Verification items for the finished model (mm, model axes). Face numbers are marked on the shaded views. A direction names the side the tool comes from. Coordinates: 2 decimals unless noted, no trailing zeros. Order: outer loops, then holes, each group sorted by start corner. A loop starts at its lowest first (then second) coordinate and runs counter-clockwise, first axis right, second up. Notation, with made-up numbers: M 20.5,-12 L 78.5,-12 A22 cw 78.5,22 Z; hole C 1,-1 d7. An arc over 180 degrees is marked long. Return JSON: item names as keys, results as strings. Group by question number.
1. Section check D-D, the plane z = 25. Record the cut outline in (x, y).
2. Material ranges on line 1 along Z through (x, y) = (-10, 3.25); line 2 along Z through (x, y) = (63, 23.5); line 3 along Z through (x, y) = (-51, 9.25), recorded low to high.
3. Set-up check for the marked faces 1 and 2: record each of +Z, -Z, +X, -X, +Y, -Y from which the full face is reachable in a straight line by a thin tool's end or side.
4. Gauge pin test, flat end, axial feed: pin 1 (12 mm diameter, centred on x = -0.5, z = -28.5, fed in from +Y). Record the tip position at first contact, or that the pin passes through.
5. Section check C-C, the plane y = 6.75. Record the cut outline in (x, z), plus the area to 3 significant figures.
6. Mould release check, pull along X, two halves, no side actions. Record for the marked faces 3, 4 and 5: +X half, -X half, draft (parallel to the pull), parting line (faces both ways), or undercut.
7. Section check B-B, the plane z = -16. Record the cut outline in (x, y).
8. Section check A-A, the plane x = 45. Record the cut outline in (y, z).
```python
from build123d import *

# Parameters (mm, degrees)
SKETCH1_W                      = 142
SKETCH1_H                      = 82
BOSS_EXTRUDE1_DEPTH            = 30
SKETCH3_W                      = 130
SKETCH3_H                      = 70
CUT_EXTRUDE1_DEPTH             = 25
FILLET1_R                      = 5
M3_CLEARANCE_HOLE1_D           = 3.2
M3_CLEARANCE_HOLE1_CSINK_D     = 3.25
M3_CLEARANCE_HOLE1_CSINK_ANGLE = 90
CUT_EXTRUDE2_REACH             = 7
CUT_EXTRUDE3_DEPTH             = 143


with BuildPart() as part:
    # Sketch1 → Boss-Extrude1 (new body)
    with BuildSketch(Plane(origin=(0, 0, 0), x_dir=(1, 0, 0), z_dir=(0, 1, 0))):
        Rectangle(SKETCH1_W, SKETCH1_H)
    extrude(amount=BOSS_EXTRUDE1_DEPTH)

    # Sketch3 → Cut-Extrude1 (cut)
    with BuildSketch(Plane(origin=(0, 30, 0), x_dir=(1, 0, 0), z_dir=(0, 1, 0))):
        Rectangle(SKETCH3_W, SKETCH3_H)
    extrude(amount=-CUT_EXTRUDE1_DEPTH, mode=Mode.SUBTRACT)

    # Fillet1
    fillet1_edges = [part.edges().sort_by_distance(p)[0] for p in [
        (71, 15, 41),
        (-71, 15, 41),
        (-71, 15, -41),
        (71, 15, -41),
    ]]
    fillet(fillet1_edges, radius=FILLET1_R)

    # M3 Clearance Hole1 (through all)
    with Locations(Plane(origin=(0, 30, 0), x_dir=(1, 0, 0), z_dir=(0, 1, 0))):
        with Locations((63, -38), (63, 38), (-63, 38), (-63, -38)):
            CounterSinkHole(M3_CLEARANCE_HOLE1_D / 2, M3_CLEARANCE_HOLE1_CSINK_D / 2, counter_sink_angle=M3_CLEARANCE_HOLE1_CSINK_ANGLE)

    # Sketch6 → Cut-Extrude2 (cut, up to next)
    with BuildSketch(Plane(origin=(0, 5, 0), x_dir=(1, 0, 0), z_dir=(0, 1, 0)), mode=Mode.PRIVATE) as cut_extrude2_sk1:
        with BuildLine():
            Line((52.5, -30), (-52.5, -30))
            ThreePointArc((-52.5, -30), (-57.5, -25), (-52.5, -20))
            Line((-52.5, -20), (52.5, -20))
            ThreePointArc((52.5, -20), (57.5, -25), (52.5, -30))
        make_face()
    cut_extrude2_tool1 = extrude(cut_extrude2_sk1.sketch, amount=-CUT_EXTRUDE2_REACH, mode=Mode.PRIVATE) & part.part
    add(cut_extrude2_tool1.solids().sort_by_distance((0, 5, 25))[0], mode=Mode.SUBTRACT)
    # Sketch6 → Cut-Extrude2 (cut, up to next)
    with BuildSketch(Plane(origin=(0, 5, 0), x_dir=(1, 0, 0), z_dir=(0, 1, 0)), mode=Mode.PRIVATE) as cut_extrude2_sk2:
        with BuildLine():
            Line((52.5, 20), (-52.5, 20))
            ThreePointArc((-52.5, 20), (-57.5, 25), (-52.5, 30))
            Line((-52.5, 30), (52.5, 30))
            ThreePointArc((52.5, 30), (57.5, 25), (52.5, 20))
        make_face()
    cut_extrude2_tool2 = extrude(cut_extrude2_sk2.sketch, amount=-CUT_EXTRUDE2_REACH, mode=Mode.PRIVATE) & part.part
    add(cut_extrude2_tool2.solids().sort_by_distance((0, 5, -25))[0], mode=Mode.SUBTRACT)

    # Sketch7 → Cut-Extrude3 (cut, through all)
    with BuildSketch(Plane(origin=(71, 0, 0), x_dir=(0, 0, -1), z_dir=(1, 0, 0))):
        with BuildLine():
            Line((-21, 21), (19, 21))
            ThreePointArc((19, 21), (25, 15), (19, 9))
            Line((19, 9), (-21, 9))
            ThreePointArc((-21, 9), (-27, 15), (-21, 21))
        make_face()
    extrude(amount=-CUT_EXTRUDE3_DEPTH, mode=Mode.SUBTRACT)


solid = part.part
```
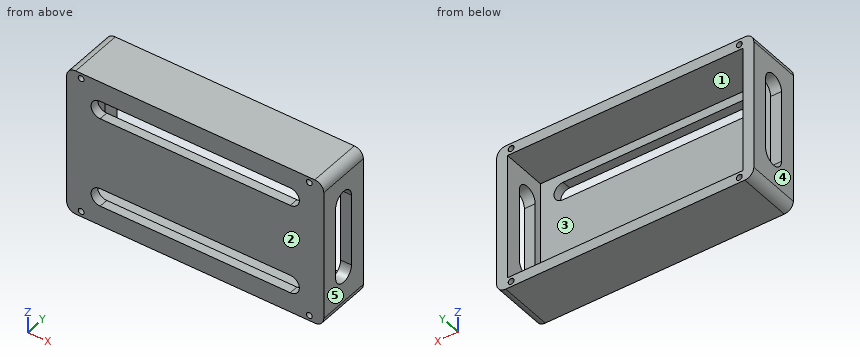
Answers follow:
{
 "1": {"outline": "M -71,0 L -57.5,0 L -57.5,5 L -65,5 L -65,10.53 L -71,10.53 Z; M -71,19.47 L -65,19.47 L -65,30 L -71,30 Z; M 57.5,0 L 71,0 L 71,10.53 L 65,10.53 L 65,5 L 57.5,5 Z; M 65,19.47 L 71,19.47 L 71,30 L 65,30 Z"},
 "2": {"line 1": "-41 to -30, -20 to 20, 30 to 41", "line 2": "-41 to -39.6, -36.4 to -35, 35 to 36.4, 39.6 to 41", "line 3": "-41 to -35, 35 to 41"},
 "3": {"face 1": "+Y", "face 2": "+Z, -Z, +X, -X, -Y"},
 "4": {"pin 1": "y = 5"},
 "5": {"outline": "M -71,-36 A5 ccw -66,-41 L 66,-41 A5 ccw 71,-36 L 71,36 A5 ccw 66,41 L -66,41 A5 ccw -71,36 Z; hole M -65,-35 L 65,-35 L 65,35 L -65,35 Z; hole C -63,-38 d3.2; hole C -63,38 d3.2; hole C 63,-38 d3.2; hole C 63,38 d3.2", "area": "2,490 mm^2"},
 "6": {"face 3": "undercut", "face 4": "-X half", "face 5": "+X half"},
 "7": {"outline": "M -71,0 L 71,0 L 71,9 L 65,9 L 65,5 L -65,5 L -65,9 L -71,9 Z; M -71,21 L -65,21 L -65,30 L -71,30 Z; M 65,21 L 71,21 L 71,30 L 65,30 Z"},
 "8": {"outline": "M 0,-41 L 30,-41 L 30,-35 L 5,-35 L 5,-30 L 0,-30 Z; M 0,-20 L 5,-20 L 5,20 L 0,20 Z; M 0,30 L 5,30 L 5,35 L 30,35 L 30,41 L 0,41 Z"}
}
